Geometry: final body of the model. Coordinates: model frame, mm. Face numbers are marked on the shaded views. A direction names the side the tool comes from. Give positions to 0.01 mm unless a question says otherwise; leave off trailing zeros. Write each loop counter-clockwise with the first axis right and the second up, starting at its lowest first coordinate (ties: lowest second). Pieces come first, ordered by that corner, then holes.
Q1. Section D-D (y = -7). Return the cut outline in (x, z).
Q2. Section A-A (y = 7). Return the cut outline in (x, z), plus the area to 3 significant figures.
Q3. Section C-C (x = 15). Return the cut outline in (y, z).
Q4. Pin query (flat end, axial travel): pin 1 Ø6 at (x, z) = (3, 23.5) entering from +Y; pin 2 Ø3 at (x, z) = (0.63, 20.75) entering from -Y. Return the tip coordinate at first contact, or that it passes through.
Q5. Reachability of the marked faces 1 and 2 from +Z, -Z, +X, -X, +Y, -Y: full face, straight path, thin tool, end or side. Return the list, or none.
Q6. Section B-B (z = 20.75). Return the cut outline in (x, y).
Q7. Line query: line 1 (Z direction, x = 32, y = -5.5); line 2 (Y direction, x = 35, z = 36). Output: solid intervals per line, ascending.
Q8. Mould query, pull axis Z, two halves, no side actions, for the marked faces 3, 4, 5 and 6. Classes: +Z half, -Z half, draft (parallel to the pull), parting line (faces both ways), or undercut.
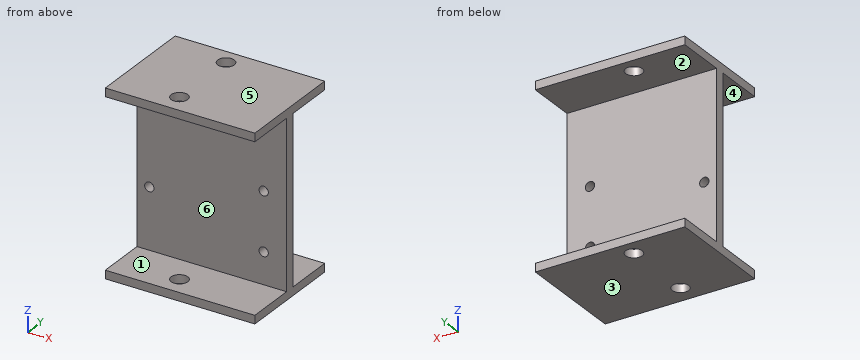
from build123d import *

# Parameters (mm, degrees)
ESQUISSE1_W             = 45
ESQUISSE1_H             = 3
BOSS_EXTRU_1_DEPTH      = 55
ESQUISSE2_R             = 1.4
ENL_V_MAT_EXTRU_1_DEPTH = 50
ESQUISSE3_W             = 45
ESQUISSE3_H             = 2.5
BOSS_EXTRU_2_DEPTH      = 15
ESQUISSE4_R             = 2.5
ENL_V_MAT_EXTRU_2_DEPTH = 65
ESQUISSE5_W             = 45
ESQUISSE5_H             = 2.5
BOSS_EXTRU_3_DEPTH      = 15
ESQUISSE6_R             = 2.5
ENL_V_MAT_EXTRU_3_DEPTH = 65


with BuildPart() as part:
    # Esquisse1 → Boss.-Extru.1 (new body)
    with BuildSketch(Plane.XY):
        with Locations((19.426229508, 2.225409836)):
            Rectangle(ESQUISSE1_W, ESQUISSE1_H)
    extrude(amount=BOSS_EXTRU_1_DEPTH)

    # Esquisse2 → Enlèv. mat.-Extru.1 (cut)
    with BuildSketch(Plane.XZ.offset(-0.725409836)):
        with Locations((0.626229508, 20.75)):
            Circle(ESQUISSE2_R)
        with Locations((35.026229508, 12)):
            Circle(ESQUISSE2_R)
        with Locations((35.026229508, 29.5)):
            Circle(ESQUISSE2_R)
    extrude(amount=-ENL_V_MAT_EXTRU_1_DEPTH, mode=Mode.SUBTRACT)

    # Esquisse3 → Boss.-Extru.2 (add)
    with BuildSketch(Plane.XZ.offset(-0.725409836)):
        with Locations((19.426229508, 53.75)):
            Rectangle(ESQUISSE3_W, ESQUISSE3_H)
        with Locations((19.426229508, 1.25)):
            Rectangle(ESQUISSE3_W, ESQUISSE3_H)
    extrude(amount=BOSS_EXTRU_2_DEPTH)

    # Esquisse4 → Enlèv. mat.-Extru.2 (cut)
    with BuildSketch(Plane.XY.offset(55)):
        with Locations((15.426229508, -8.274590164)):
            Circle(ESQUISSE4_R)
    extrude(amount=-ENL_V_MAT_EXTRU_2_DEPTH, mode=Mode.SUBTRACT)

    # Esquisse5 → Boss.-Extru.3 (add)
    with BuildSketch(Plane(origin=(0, 3.725409836, 0), x_dir=(1, 0, 0), z_dir=(0, 1, 0))):
        with Locations((19.426229508, -53.75)):
            Rectangle(ESQUISSE5_W, ESQUISSE5_H)
        with Locations((19.426229508, -1.25)):
            Rectangle(ESQUISSE5_W, ESQUISSE5_H)
    extrude(amount=BOSS_EXTRU_3_DEPTH)

    # Esquisse6 → Enlèv. mat.-Extru.3 (cut)
    with BuildSketch(Plane.XY.offset(55)):
        with Locations((15.426229508, 13.725409836)):
            Circle(ESQUISSE6_R)
    extrude(amount=-ENL_V_MAT_EXTRU_3_DEPTH, mode=Mode.SUBTRACT)


solid = part.part
Computed:
1. outline: (-3.07, 0) - (13.28, 0) - (13.28, 2.5) - (-3.07, 2.5) - close; (-3.07, 52.5) - (13.28, 52.5) - (13.28, 55) - (-3.07, 55) - close; (17.58, 0) - (41.93, 0) - (41.93, 2.5) - (17.58, 2.5) - close; (17.58, 52.5) - (41.93, 52.5) - (41.93, 55) - (17.58, 55) - close
2. outline: (-3.07, 0) - (41.93, 0) - (41.93, 2.5) - (-3.07, 2.5) - close; (-3.07, 52.5) - (41.93, 52.5) - (41.93, 55) - (-3.07, 55) - close
2. area: 225 mm2
3. outline: (-14.27, 0) - (-10.74, 0) - (-10.74, 2.5) - (-14.27, 2.5) - close; (-14.27, 52.5) - (-10.74, 52.5) - (-10.74, 55) - (-14.27, 55) - close; (-5.81, 0) - (11.26, 0) - (11.26, 2.5) - (3.73, 2.5) - (3.73, 52.5) - (11.26, 52.5) - (11.26, 55) - (-5.81, 55) - (-5.81, 52.5) - (0.73, 52.5) - (0.73, 2.5) - (-5.81, 2.5) - close; (16.19, 0) - (18.73, 0) - (18.73, 2.5) - (16.19, 2.5) - close; (16.19, 52.5) - (18.73, 52.5) - (18.73, 55) - (16.19, 55) - close
4. pin 1: stops at y = 3.73
4. pin 2: stops at y = 0.73
5. face 1: +X, -X, -Y
5. face 2: +X, -X, +Y
6. outline: (-3.07, 0.73) - (-0.77, 0.73) - (-0.77, 3.73) - (-3.07, 3.73) - close; (2.03, 0.73) - (41.93, 0.73) - (41.93, 3.73) - (2.03, 3.73) - close
7. line 1: z = 0 to 2.5, 52.5 to 55
7. line 2: y = 0.73 to 3.73
8. face 3: -Z half
8. face 4: undercut
8. face 5: +Z half
8. face 6: undercut
